```python
from build123d import *

# Parameters (mm, degrees)
F1_DEPTH      = 3.175
F1_DEPTH_BACK = 30.1498
F2_DEPTH      = 25.4
F3_DEPTH      = 25.4
F4_START      = -7.9248
F4_DEPTH      = 9.8298
F5_DEPTH      = 52.3748


with BuildPart() as f1:
    # F0 (on Top) → F1 (new body, two sides)
    with BuildSketch(Plane.XY) as f1_sk:
        with BuildLine():
            Line((-22.225, 0), (-19.05, 0))
            ThreePointArc((-19.05, 0), (-19.9154840123, 6.5740037456), (-22.4529547439, 12.7))
            ThreePointArc((-22.4529547439, 12.7), (-31.75, 21.9970452561), (-44.45, 25.4))
            Line((-44.45, 25.4), (-44.45, 22.225))
            ThreePointArc((-44.45, 22.225), (-28.7345517881, 15.7154482119), (-22.225, 0))
        make_face()
        with BuildLine():
            ThreePointArc((-22.4529547439, -12.7), (-19.9154840123, -6.5740037456), (-19.05, 0))
            Line((-19.05, 0), (-22.225, 0))
            ThreePointArc((-22.225, 0), (-60.1654482119, -15.7154482119), (-44.45, 22.225))
            Line((-44.45, 22.225), (-44.45, 25.4))
            ThreePointArc((-44.45, 25.4), (-66.4470452561, -12.7), (-22.4529547439, -12.7))
        make_face()
        with BuildLine():
            ThreePointArc((-44.45, 22.225), (-60.1654482119, -15.7154482119), (-22.225, 0))
            Line((-22.225, 0), (-31.75, 0))
            ThreePointArc((-31.75, 0), (-53.4302561211, -8.9802561211), (-44.45, 12.7))
            Line((-44.45, 12.7), (-44.45, 22.225))
        make_face()
        with BuildLine():
            Line((-31.75, 0), (-22.225, 0))
            ThreePointArc((-22.225, 0), (-28.7345517881, 15.7154482119), (-44.45, 22.225))
            Line((-44.45, 22.225), (-44.45, 12.7))
            ThreePointArc((-44.45, 12.7), (-35.4697438789, 8.9802561211), (-31.75, 0))
        make_face()
    extrude(amount=F1_DEPTH)
    extrude(f1_sk.sketch, amount=-F1_DEPTH_BACK)



with BuildPart() as f2:
    # F0 (on Top) → F2 (new body)
    with BuildSketch(Plane.XY):
        with BuildLine():
            ThreePointArc((46.5639319141, 45.1555555556), (52.8217153018, 29.3389400327), (56.3531249516, 12.7))
            ThreePointArc((56.3531249516, 12.7), (56.9505855384, 6.3624879144), (57.15, 0))
            ThreePointArc((57.15, 0), (56.9505855384, -6.3624879144), (56.3531249516, -12.7))
            ThreePointArc((56.3531249516, -12.7), (55.6033339134, -17.6604182514), (54.6095979732, -22.5777777778))
            ThreePointArc((54.6095979732, -22.5777777778), (64.1698254977, -37.7824497467), (79.3744974665, -28.2222222222))
            ThreePointArc((79.3744974665, -28.2222222222), (81.6634026015, 14.9803098855), (69.3174148927, 56.4444444444))
            ThreePointArc((69.3174148927, 56.4444444444), (54.7801695925, 63.1004559127), (45.25211394, 50.2610577545))
            Line((45.25211394, 50.2610577545), (46.5639319141, 45.1555555556))
        make_face()
        with BuildLine():
            ThreePointArc((60.8008228466, -23.9888888889), (62.823083358, -12.0701320149), (63.5, 0))
            ThreePointArc((63.5, 0), (60.6504663929, 24.6392870025), (52.2523026588, 47.9777777778))
            ThreePointArc((52.2523026588, 47.9777777778), (55.1184511812, 56.4883707446), (63.629044148, 53.6222222222))
            ThreePointArc((63.629044148, 53.6222222222), (75.3577324715, 14.2312943912), (73.1832725932, -26.8111111111))
            ThreePointArc((73.1832725932, -26.8111111111), (65.5809366088, -31.5912248733), (60.8008228466, -23.9888888889))
        make_face(mode=Mode.SUBTRACT)
    extrude(amount=-F2_DEPTH)


with BuildPart() as f1_1:
    add(f1.part)

    add(f2.part)  # F3 merges F2
    # F0 (on Top) → F3 (join)
    with BuildSketch(Plane.XY):
        with BuildLine():
            Line((-5.5499, 0), (-19.05, 0))
            ThreePointArc((-19.05, 0), (-19.9154840123, -6.5740037456), (-22.4529547439, -12.7))
            Line((-22.4529547439, -12.7), (0, -12.7))
            Line((0, -12.7), (0, -5.5499))
            ThreePointArc((0, -5.5499), (-3.9243719249, -3.9243719249), (-5.5499, 0))
        make_face()
        with BuildLine():
            ThreePointArc((-22.4529547439, 12.7), (-19.9154840123, 6.5740037456), (-19.05, 0))
            Line((-19.05, 0), (-5.5499, 0))
            ThreePointArc((-5.5499, 0), (-3.9243719249, 3.9243719249), (0, 5.5499))
            Line((0, 5.5499), (0, 12.7))
            Line((0, 12.7), (-22.4529547439, 12.7))
        make_face()
        with BuildLine():
            Line((0, 12.7), (0, 5.5499))
            Line((0, 5.5499), (38.1, 5.5499))
            ThreePointArc((38.1, 5.5499), (42.0243719249, 3.9243719249), (43.6499, 0))
            Line((43.6499, 0), (57.15, 0))
            ThreePointArc((57.15, 0), (56.9505855384, 6.3624879144), (56.3531249516, 12.7))
            Line((56.3531249516, 12.7), (0, 12.7))
        make_face()
        with BuildLine():
            Line((38.1, -5.5499), (0, -5.5499))
            Line((0, -5.5499), (0, -12.7))
            Line((0, -12.7), (56.3531249516, -12.7))
            ThreePointArc((56.3531249516, -12.7), (56.9505855384, -6.3624879144), (57.15, 0))
            Line((57.15, 0), (43.6499, 0))
            ThreePointArc((43.6499, 0), (42.0243719249, -3.9243719249), (38.1, -5.5499))
        make_face()
    extrude(amount=-F3_DEPTH)

    # F0 (on Top) → F4 (join)
    with BuildSketch(Plane.XY.offset(F4_START)):
        with BuildLine():
            ThreePointArc((-44.45, 25.4), (-31.75, 21.9970452561), (-22.4529547439, 12.7))
            Line((-22.4529547439, 12.7), (0, 12.7))
            Line((0, 12.7), (56.3531249516, 12.7))
            ThreePointArc((56.3531249516, 12.7), (52.8217153018, 29.3389400327), (46.5639319141, 45.1555555556))
            Line((46.5639319141, 45.1555555556), (45.25211394, 50.2610577545))
            ThreePointArc((45.25211394, 50.2610577545), (43.9347743486, 46.1118478743), (40.2548039053, 43.7860912739))
            Line((40.2548039053, 43.7860912739), (-44.45, 25.4))
        make_face()
    extrude(amount=-F4_DEPTH)

    # F0 (on Top) → F5 (join)
    with BuildSketch(Plane.XY):
        with BuildLine():
            ThreePointArc((-44.45, 22.225), (-60.1654482119, -15.7154482119), (-22.225, 0))
            Line((-22.225, 0), (-31.75, 0))
            ThreePointArc((-31.75, 0), (-53.4302561211, -8.9802561211), (-44.45, 12.7))
            Line((-44.45, 12.7), (-44.45, 22.225))
        make_face()
        with BuildLine():
            Line((-31.75, 0), (-22.225, 0))
            ThreePointArc((-22.225, 0), (-28.7345517881, 15.7154482119), (-44.45, 22.225))
            Line((-44.45, 22.225), (-44.45, 12.7))
            ThreePointArc((-44.45, 12.7), (-35.4697438789, 8.9802561211), (-31.75, 0))
        make_face()
    extrude(amount=-F5_DEPTH)


solid = f1_1.part
```
Geometry: final body of the model. Coordinates: model frame, mm. A direction names the side the tool comes from. Give positions to 0.01 mm unless a question says otherwise; leave off trailing zeros. Write each loop counter-clockwise with the first axis right and the second up, starting at its lowest first coordinate (ties: lowest second). Pieces come first, ordered by that corner, then holes.
1. Section query B-B, the plane y = -14.5. Return loops of the section in (x, z) (1 decimal).
2. Draft query along Y for faces 1 (the cylindrical face through (81.734, 14.376, -12.522)), 2 (the flat face through (-1.505, 34.722, -12.771)), 3 (the cylindrical face through (65.72, -31.62, -12.52)), 4 (the cylindrical face through (75.288, 14.805, -12.522)). Return one class per face: released by +Y, released by -Y, zero draft, split by the parting line, or undercut.
3. Section query D-D, the plane z = -35.5. Return loops of the section in (x, y) (3 decimals).
4. Line query: probe 1 along Y at (x, z) = (31, -6); probe 2 along X at (y, z) = (-18, -8.5); probe 3 along Y at (x, z) = (-44.45, -9.5). Output: solid intervals per line, ascending.
5. Section query A-A, the plane z = -20.5. Return loops of the section in (x, y).
6. Pin query (flat end, axial travel): P1, Ø2, axis at x = -21, z = -20.5, coming from the +Y side; P2, Ø20.5, axis at x = 34.5, y = 2, coming from the +Z side; P3, Ø20.5, axis at x = 13, y = -2.5, coming from the -Z side. Return the tip coordinate at first contact, or that it passes through.
7. Section query C-C, the plane y = 19.5. Return loops of the section in (x, z) (3 decimals), then the cut area to 3 significant figures.
8. Reachability of faces 5 (the cylindrical face through (52.75, 29.57, -3.91)), 6 (the flat face through (19, -5.55, -13)), 7 (the flat face through (16, 28, -17.755)) from +Z, -Z, +X, -X, +Y, -Y: full face, straight path, thin tool, end or side. Return the list, or none.
Computed:
1. outline: (-65.3, -30.1) - (-61.3, -30.1) - (-61.3, -52.4) - (-27.6, -52.4) - (-27.6, -30.1) - (-23.6, -30.1) - (-23.6, 3.2) - (-65.3, 3.2) - close; (56.1, -25.4) - (62.5, -25.4) - (62.5, 0) - (56.1, 0) - close; (75.3, -25.4) - (81.7, -25.4) - (81.7, 0) - (75.3, 0) - close
2. face 1: split by the parting line
2. face 2: released by +Y
2. face 3: undercut
2. face 4: undercut
3. outline: circle Ø44.45 at (-44.45, 0); hole circle Ø25.4 at (-44.45, 0)
4. probe 1: y = -12.7 to -5.55, 5.55 to 12.7
4. probe 2: x = -62.37 to -26.53, 55.54 to 61.99, 74.85 to 81.27
4. probe 3: y = -25.4 to -12.7, 12.7 to 25.4
5. outline: (-22.45, -12.7) - (56.35, -12.7) arc R101.6 cw to (54.61, -22.58) arc R12.7 ccw to (79.37, -28.22) arc R127 ccw to (69.32, 56.44) arc R12.7 ccw to (45.25, 50.26) - (46.56, 45.16) arc R101.6 cw to (56.35, 12.7) - (-22.45, 12.7) arc R25.4 ccw (long way) to start; hole circle Ø25.4 at (-44.45, 0); hole (0, -5.55) - (38.1, -5.55) arc R5.55 ccw to (38.1, 5.55) - (0, 5.55) arc R5.55 ccw to start; hole (52.25, 47.98) arc R107.95 cw to (60.8, -23.99) arc R6.35 ccw to (73.18, -26.81) arc R120.65 ccw to (63.63, 53.62) arc R6.35 ccw to start
6. P1: stops at y = 12.7
6. P2: stops at z = 0
6. P3: stops at z = -25.4
7. outline: (-60.726, -30.15) - (-55.113, -30.15) - (-55.113, -52.375) - (-33.787, -52.375) - (-33.787, -30.15) - (-28.174, -30.15) - (-28.174, -17.755) - (55.261, -17.755) - (55.261, -25.4) - (61.724, -25.4) - (61.724, 0) - (55.261, 0) - (55.261, -7.925) - (-28.174, -7.925) - (-28.174, 3.175) - (-60.726, 3.175) - close; (74.614, -25.4) - (81.044, -25.4) - (81.044, 0) - (74.614, 0) - close
7. area: 2,710 mm2
8. face 5: +Z
8. face 6: +Z, -Z
8. face 7: -Z
